from build123d import *

# Parameters (mm, degrees)
F1_DEPTH = 25.4


with BuildPart() as f1:
    # F0 (on Right) → F1 (new body)
    with BuildSketch(Plane.YZ):
        with BuildLine():
            ThreePointArc((-10.843395, 99.24675), (-30.582903, 89.831488), (-35.688344, 68.565793))
            Line((-35.688344, 68.565793), (-5.243084, -74.667893))
            Line((-5.243084, -74.667893), (96.356916, -74.667893))
            Line((96.356916, -74.667893), (96.356916, -61.967893))
            ThreePointArc((96.356916, -61.967893), (88.917428, -44.007381), (70.956916, -36.567893))
            Line((70.956916, -36.567893), (46.178202, -36.567893))
            ThreePointArc((46.178202, -36.567893), (30.193464, -30.907401), (21.333253, -16.44885))
            Line((21.333253, -16.44885), (-3.258606, 99.24675))
            Line((-3.258606, 99.24675), (-10.843395, 99.24675))
        make_face()
    extrude(amount=F1_DEPTH)


solid = f1.part
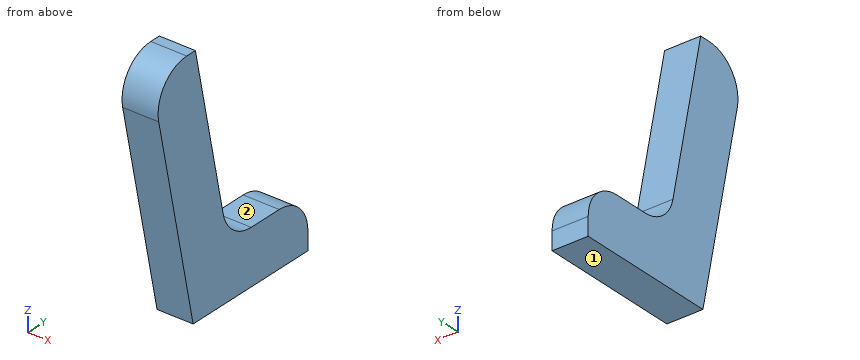
Could you check a few things on this model? Use its own coordinates, in mm. Face numbers are marked on the shaded views. A direction names the side the tool comes from. Give positions to 0.01 mm unless a question says otherwise; leave off trailing zeros. Order: outer loops, then holes, each group sorted by start corner. A loop starts at its lowest first (then second) coordinate and runs counter-clockwise, first axis right, second up. Notation, with made-up numbers: (59, 86.5) -> (89, 86.5) arc R30 cw to (89, 122.5) -> close; hole circle Ø3 at (-20.5, -23). An arc over 180 degrees is marked (long way). Answer in a Markdown table with one row per item. Add a question column.
Item 1: Imagine slicing it at B-B (z = 80). List the corners of the cut face in (x, y) for me, and give its area (3 significant figures).
Item 2: Please list where these lines run through material, in increasing order: probe 1 along Z at (x, y) = (8.25, 42); probe 2 along Z at (x, y) = (5.5, 59); probe 3 along Y at (x, z) = (20.5, 85).
Item 3: For the marked faces 1 and 2, which set-ups out of +Z, -Z, +X, -X, +Y, -Y let a thin tool reach every point of the face, with its end or its side?
Item 4: Imagine slicing it at A-A (x = 23). List the corners of the cut face in (y, z) for me, and give its area (3 significant figures).
Item 5: I'm going to push flat-ended pins straight in: P1, Ø4, axis at x = 12.5, y = -15, coming from the +Z side; P2, Ø10, axis at x = 22, z = -13, coming from the -Y side; P3, Ø4, axis at x = 18, z = 37.5, coming from the +Y side. Where does each tip first touch, or does it pass through?
Item 6: Imagine slicing it at C-C (y = 12). List the corners of the cut face in (x, z) for me.
Result:
| question | item | result |
|---|---|---|
| 1 | outline | (0, -35.49) -> (25.4, -35.49) -> (25.4, 0.83) -> (0, 0.83) -> close |
| 1 | area | 923 mm2 |
| 2 | probe 1 | -74.67 to -36.22 |
| 2 | probe 2 | -74.67 to -36.57 |
| 2 | probe 3 | -33.66 to -0.23 |
| 3 | face 1 | -Z, +X, -X, +Y, -Y |
| 3 | face 2 | +Z, +X, -X, +Y |
| 4 | outline | (-35.69, 68.57) -> (-5.24, -74.67) -> (96.36, -74.67) -> (96.36, -61.97) arc R25.4 ccw to (70.96, -36.57) -> (46.18, -36.57) arc R25.4 cw to (21.33, -16.45) -> (-3.26, 99.25) -> (-10.84, 99.25) arc R25.4 ccw to start |
| 4 | area | 9,040 mm2 |
| 5 | P1 | z = 99.16 |
| 5 | P2 | y = -19.41 |
| 5 | P3 | y = 10.29 |
| 6 | outline | (0, -74.67) -> (25.4, -74.67) -> (25.4, 27.46) -> (0, 27.46) -> close |
